The drawing under review shows one solid part. Ordinate dimensions are in mm from its lowest x, y, z. Coordinates: 2 decimals unless noted, no trailing zeros. Loops run counter-clockwise (first coordinate to the right, second up) from the corner with the lowest first, then second, coordinate; pieces in that order, holes last. Notation, with made-up numbers: (82.5, 49.5) - (118.5, 49.5) arc R12 ccw to (118.5, 57.5) - close; hole circle Ø3 at (-37, 13). An arc over 180 degrees is marked (long way). Answer as a JSON object with one key per item and string values. Group by question number.
Item 1: We need section A-A (y = 3.75). Give the boundary of the cut face in (x, z).
Item 2: Clearance check with flat-ended pins moving along their axes: pin 1 (0.8 mm diameter, centred on x = 20, z = 8, fed in from +Y); pin 2 (4 mm diameter, centred on x = 19.5, y = 4.5, fed in from +Z). State where each tip first meets the part, or that it passes through.
Item 3: We need section C-C (z = 4). Give the boundary of the cut face in (x, y).
Item 4: We need section B-B (x = 22). Give the boundary of the cut face in (y, z).
Item 5: To check wall thickness, follow line 1 (X direction, y = 7.25, z = 5); line 2 (Z direction, x = 9.5, y = 5.75); line 3 (Y direction, x = 20.25, z = 12.5). State the ranges of each line that lie inside material, in increasing order.
Item 6: We need section D-D (y = 2). Give the boundary of the cut face in (x, z), then the cut area to 3 significant figures.
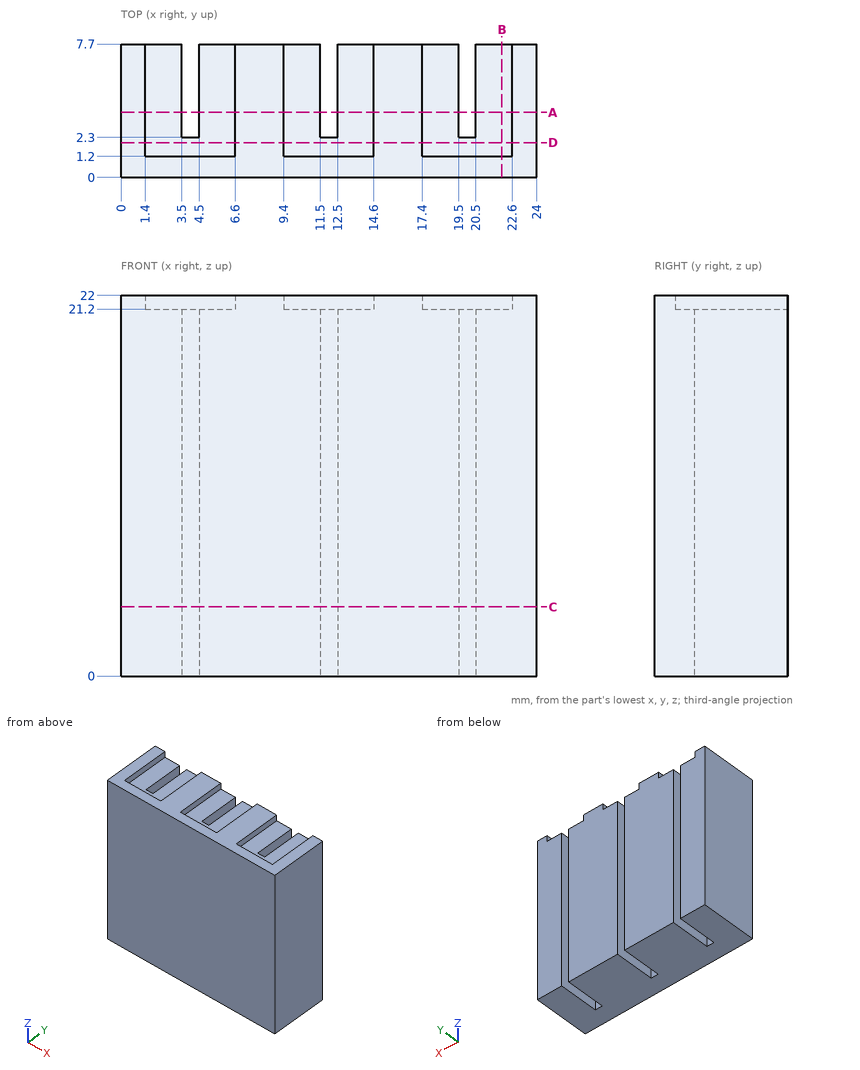
Check sheet entries:
{
 "1": {"outline": "(0, 0) - (3.5, 0) - (3.5, 21.2) - (1.4, 21.2) - (1.4, 22) - (0, 22) - close; (4.5, 0) - (11.5, 0) - (11.5, 21.2) - (9.4, 21.2) - (9.4, 22) - (6.6, 22) - (6.6, 21.2) - (4.5, 21.2) - close; (12.5, 0) - (19.5, 0) - (19.5, 21.2) - (17.4, 21.2) - (17.4, 22) - (14.6, 22) - (14.6, 21.2) - (12.5, 21.2) - close; (20.5, 0) - (24, 0) - (24, 22) - (22.6, 22) - (22.6, 21.2) - (20.5, 21.2) - close"},
 "2": {"pin 1": "stops at y = 2.3", "pin 2": "stops at z = 21.2"},
 "3": {"outline": "(0, 0) - (24, 0) - (24, 7.7) - (20.5, 7.7) - (20.5, 2.3) - (19.5, 2.3) - (19.5, 7.7) - (12.5, 7.7) - (12.5, 2.3) - (11.5, 2.3) - (11.5, 7.7) - (4.5, 7.7) - (4.5, 2.3) - (3.5, 2.3) - (3.5, 7.7) - (0, 7.7) - close"},
 "4": {"outline": "(0, 0) - (7.7, 0) - (7.7, 21.2) - (1.2, 21.2) - (1.2, 22) - (0, 22) - close"},
 "5": {"line 1": "x = 0 to 3.5, 4.5 to 11.5, 12.5 to 19.5, 20.5 to 24", "line 2": "z = 0 to 21.2", "line 3": "y = 0 to 2.3"},
 "6": {"outline": "(0, 0) - (24, 0) - (24, 22) - (22.6, 22) - (22.6, 21.2) - (17.4, 21.2) - (17.4, 22) - (14.6, 22) - (14.6, 21.2) - (9.4, 21.2) - (9.4, 22) - (6.6, 22) - (6.6, 21.2) - (1.4, 21.2) - (1.4, 22) - (0, 22) - close", "area": "516 mm2"}
}
